Verification items for the finished model (mm, model axes). Coordinates: 2 decimals unless noted, no trailing zeros. Order: outer loops, then holes, each group sorted by start corner. A loop starts at its lowest first (then second) coordinate and runs counter-clockwise, first axis right, second up. Notation, with made-up numbers: (36, 0.5) -> (85, 0.5) arc R11 ccw to (85, 10.5) -> close; hole circle Ø6 at (24, -3.75). An arc over 180 degrees is marked (long way). Write item = value, one per line. Start each with the question number.
1. Cross-section at B-B on x = 4. Record the cut outline in (y, z).
2. Cross-section at A-A on y = 13. Record the cut outline in (x, z), plus the area to 3 significant figures.
3. Thickness scan on line 1 along Y through (x, z) = (13.5, 0.65); line 2 along Y through (x, z) = (-35, 0.3); line 3 along X through (y, z) = (-7, 0.3). Record the ranges inside material, lowest first. Write a range as from..to.
4. Cross-section at C-C on z = 0.8. Record the cut outline in (x, y).
from build123d import *

# Parameters (mm, degrees)
PAD_DEPTH = 1.6


with BuildPart() as part:
    # Sketch → Pad (new body)
    with BuildSketch(Plane.XY):
        with BuildLine():
            ThreePointArc((28.180802, 9.808205), (13.613929, 24.235706), (-6.303954, 19.375204))
            ThreePointArc((-6.303954, 19.375204), (-16.710147, 21.253139), (-25.769512, 15.799387))
            ThreePointArc((-25.769512, 15.799387), (-37.287949, 11.865644), (-40, 0))
            ThreePointArc((-19.819198, -15.191795), (-27.370121, -4.222451), (-40, 0))
            ThreePointArc((-8.038434, -24.865429), (-12.432827, -18.206764), (-19.819198, -15.191795))
            ThreePointArc((6.230488, -9.200613), (-5.240972, -13.082492), (-8.038434, -24.865429))
            ThreePointArc((25.696046, -5.624796), (15.289853, -3.746861), (6.230488, -9.200613))
            ThreePointArc((40, 0), (32.314926, -1.456724), (25.696046, -5.624796))
            ThreePointArc((40, 0), (35.621137, 6.748689), (28.180802, 9.808205))
        make_face()
        with BuildLine():
            ThreePointArc((-25.14228, 14.122309), (-35.472766, 11.572036), (-38.810792, 1.468551))
            ThreePointArc((-18.675961, -13.821187), (-26.392811, -3.080893), (-38.810792, 1.468551))
            ThreePointArc((-9.72633, -18.745392), (-13.769068, -15.497999), (-18.675961, -13.821187))
            ThreePointArc((5.618325, -7.593849), (-4.230442, -10.174814), (-9.72633, -18.745392))
            ThreePointArc((25.494301, -3.800154), (14.906517, -2.292583), (5.618325, -7.593849))
            ThreePointArc((37.889878, 1.400834), (31.294602, -0.252324), (25.494301, -3.800154))
            ThreePointArc((37.889878, 1.400834), (33.464455, 6.469882), (27.006338, 8.359943))
            ThreePointArc((27.006338, 8.359943), (13.164593, 22.803643), (-6.112904, 17.456446))
            ThreePointArc((-6.112904, 17.456446), (-16.329844, 19.797437), (-25.14228, 14.122309))
        make_face(mode=Mode.SUBTRACT)
    extrude(amount=PAD_DEPTH)


solid = part.part
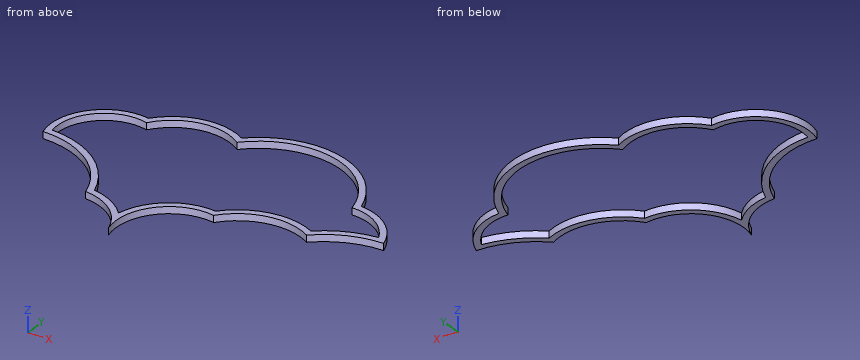
Worked out:
q1.outline = (-9, 0) -> (-7.5, 0) -> (-7.5, 1.6) -> (-9, 1.6) -> close; (23.09, 0) -> (24.62, 0) -> (24.62, 1.6) -> (23.09, 1.6) -> close
q2.outline = (-36.12, 0) -> (-33.55, 0) -> (-33.55, 1.6) -> (-36.12, 1.6) -> close; (25.3, 0) -> (26.97, 0) -> (26.97, 1.6) -> (25.3, 1.6) -> close
q2.area = 6.81 mm²
q3.line_1 = -4.19..-2.63, 22.71..24.27
q3.line_2 = -0.6..0.94, 11.99..13.86
q3.line_3 = -24.35..-22.39, 6.17..8.37
q4.outline = (-40, 0) arc R21 cw to (-19.82, -15.19) arc R13.5 cw to (-8.04, -24.87) arc R12.5 cw to (6.23, -9.2) arc R15 cw to (25.7, -5.62) arc R21 cw to (40, 0) arc R13.5 ccw to (28.18, 9.81) arc R21 ccw to (-6.3, 19.38) arc R15 ccw to (-25.77, 15.8) arc R12.5 ccw to start; hole (-38.81, 1.47) arc R22.5 cw to (-18.68, -13.82) arc R15 cw to (-9.73, -18.75) arc R14 cw to (5.62, -7.59) arc R16.5 cw to (25.49, -3.8) arc R22.5 cw to (37.89, 1.4) arc R12 ccw to (27.01, 8.36) arc R19.5 ccw to (-6.11, 17.46) arc R13.5 ccw to (-25.14, 14.12) arc R11 ccw to start
